Input: dimensioned drawing with shaded views. Units: mm. Origin: part minimum x, y, z. A direction names the side the tool comes from. Give positions to 0.01 mm unless a question says otherwise; leave off trailing zeros. Loops run counter-clockwise (first coordinate to the right, second up) from the corner with the lowest first, then second, coordinate; pieces in that order, holes last. Notation, with made-up numbers: M 54,80.25 L 96,80.25 A25 cw 96,103.25 Z; hole C -8.5,78 d1. An arc over 180 degrees is marked long. One line per question, with ' | ' between items. Start each with the question number.
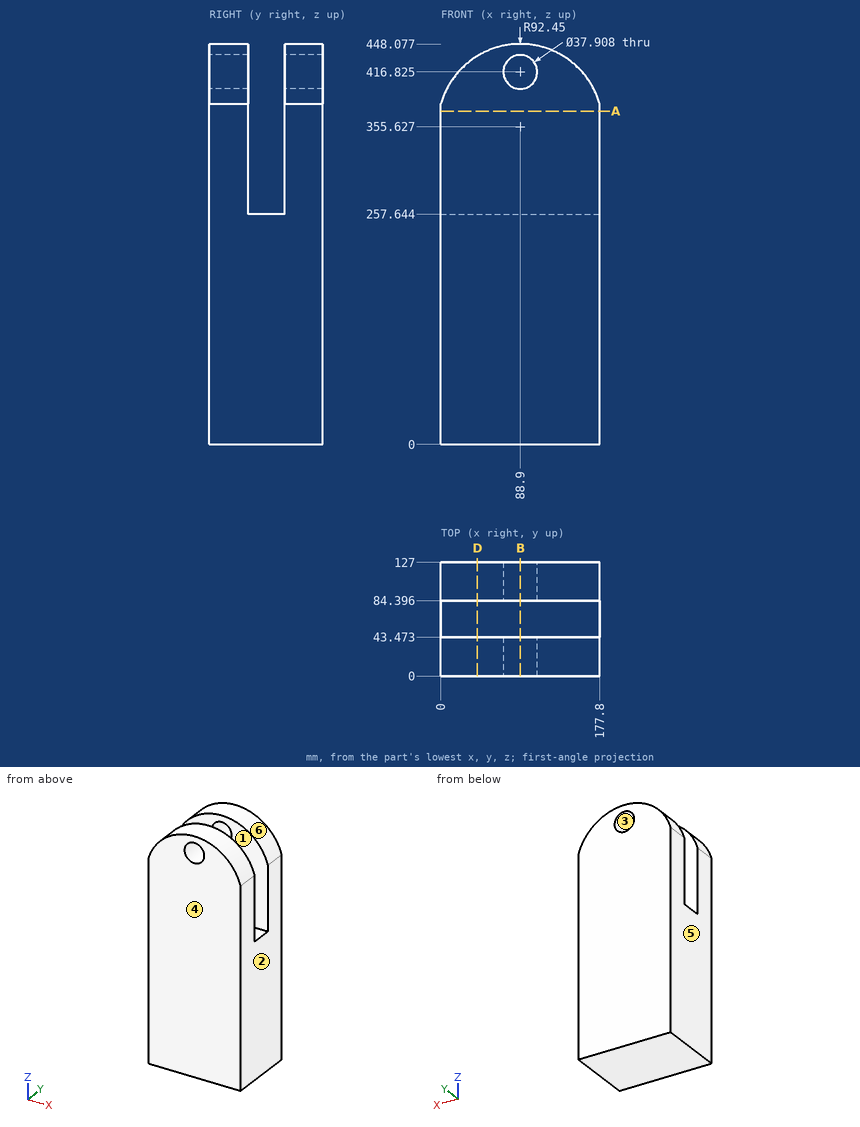
Q1. Set-up query: the marked faces 1 and 2. Return all of +Z, -Z, +X, -X, +Y, -Y with unobstructed straight access to the full face (end or side cutting, diameter ignored); none if empty.
Q2. Contact query for flat-ended pins moving along their axis: pin 1 (2 mm diameter, centred on x = 20.5, y = 32.5, fed in from +Z) (1 decimal); pin 2 (10 mm diameter, centred on x = 32, y = 107, fed in from +Z) (1 decimal); pin 3 (6 mm diameter, centred on x = 40, y = 93, fed in from +Z). Output: stop coordinate, or through.
Q3. Section A-A, the plane z = 373. Output: boundary loops of the cut face in (x, y) (1 decimal).
Q4. Section D-D, the plane x = 41. Output: boundary loops of the cut face in (y, z) (1 decimal).
Q5. Section B-B, the plane x = 88.9. Output: boundary loops of the cut face in (y, z) (1 decimal), plus the area to 4 significant figures.
Q6. Draft query along X for the marked faces 3, 4, 5 and 6. Return one class per face: released by +X, released by -X, zero draft, split by the parting line, or undercut.
Q7. Material intervals for L1, parallel to Y at x = 135, z = 281 (1 decimal); L2, parallel to Z at x = 88.9, y = 31; L3, parallel to Z at x = 103.5, y = 110 (1 decimal), sorted ascending.
Model answer:
1) face 1: +Z, +X, -X | face 2: +Z, -Z, +X, +Y, -Y
2) pin 1: stops at z = 418.9 | pin 2: stops at z = 432.1 | pin 3: stops at z = 435.88
3) outline: M 0,0 L 177.8,0 L 177.8,43.5 L 0,43.5 Z; M 0,84.4 L 177.8,84.4 L 177.8,127 L 0,127 Z
4) outline: M 0,0 L 127,0 L 127,434.7 L 84.4,434.7 L 84.4,257.6 L 43.5,257.6 L 43.5,434.7 L 0,434.7 Z
5) outline: M 0,0 L 127,0 L 127,397.9 L 84.4,397.9 L 84.4,257.6 L 43.5,257.6 L 43.5,397.9 L 0,397.9 Z; M 0,435.8 L 43.5,435.8 L 43.5,448.1 L 0,448.1 Z; M 84.4,435.8 L 127,435.8 L 127,448.1 L 84.4,448.1 Z | area: 45,850 mm^2
6) face 3: undercut | face 4: zero draft | face 5: released by -X | face 6: split by the parting line
7) L1: y = 0 to 43.5, 84.4 to 127 | L2: z = 0 to 397.87, 435.78 to 448.08 | L3: z = 0 to 404.7, 428.9 to 446.9
